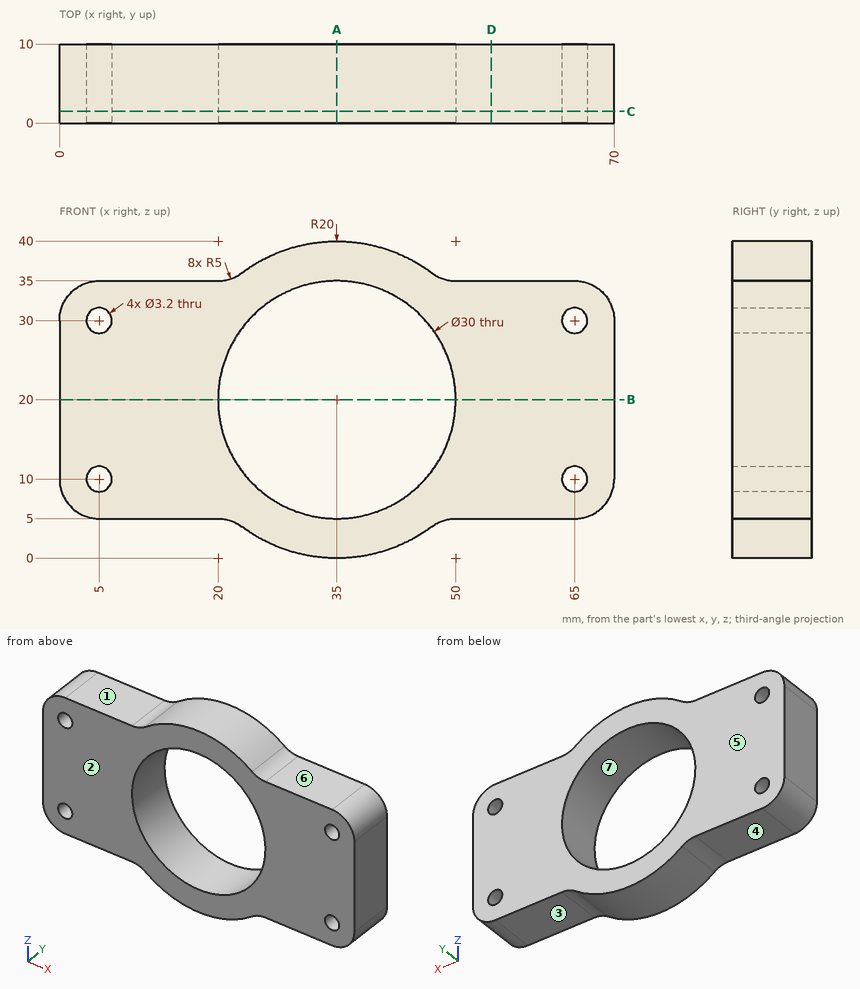
Input: dimensioned drawing with shaded views. Units: mm. Origin: part minimum x, y, z. A direction names the side the tool comes from. Coordinates: 2 decimals unless noted, no trailing zeros. Order: outer loops, then holes, each group sorted by start corner. A loop starts at its lowest first (then second) coordinate and runs counter-clockwise, first axis right, second up. Notation, with made-up numbers: (86, 71) - (143, 71) arc R30 ccw to (143, 104) - close; hole circle Ø11 at (59, 21.25). An arc over 180 degrees is marked (long way). One line per item, written item: value.
1) Reachability of the marked faces 1, 2 and 3 from +Z, -Z, +X, -X, +Y, -Y: full face, straight path, thin tool, end or side. Return the list, or none.
Computed values:
face 1: +Z, -X, +Y, -Y
face 2: +Z, -Z, +X, -X, -Y
face 3: -Z, +X, +Y, -Y
2) Contact query for a flat-ended pin moving along its axis: pin 1 (5 mm diameter, centred on x = 10.5, y = 5.5, fed in from +Z). Output: stop coordinate, or through.
Computed values:
pin 1: stops at z = 35
3) Cut plane D-D on x = 54.5. Output: boundary loops of the cut face in (y, z).
Computed values:
outline: (0, 5) - (10, 5) - (10, 35) - (0, 35) - close
4) Cut plane B-B on z = 20. Output: boundary loops of the cut face in (x, y).
Computed values:
outline: (0, 0) - (20, 0) - (20, 10) - (0, 10) - close; (50, 0) - (70, 0) - (70, 10) - (50, 10) - close
5) Mould query, pull axis Z, two halves, no side actions, for the marked faces 4, 5, 6 and 7. Classes: released by +Z, released by -Z, zero draft, split by the parting line, or undercut.
Computed values:
face 4: released by -Z
face 5: zero draft
face 6: released by +Z
face 7: undercut
6) Ray query, line 1 (X direction, y = 5.75, z = 10); line 2 (Z direction, x = 5, y = 3.5); line 3 (X direction, y = 2.75, z = 20). Return the intervals inside material, ascending. Write a range as [from, to].
Computed values:
line 1: x = [0, 3.4], [6.6, 23.82], [46.18, 63.4], [66.6, 70]
line 2: z = [5, 8.4], [11.6, 28.4], [31.6, 35]
line 3: x = [0, 20], [50, 70]
7) Cut plane C-C on y = 1.5. Output: boundary loops of the cut face in (x, z), plus the area to 3 significant figures.
Computed values:
outline: (0, 10) arc R5 ccw to (5, 5) - (20, 5) arc R5 cw to (23, 4) arc R20 ccw to (47, 4) arc R5 cw to (50, 5) - (65, 5) arc R5 ccw to (70, 10) - (70, 30) arc R5 ccw to (65, 35) - (50, 35) arc R5 cw to (47, 36) arc R20 ccw to (23, 36) arc R5 cw to (20, 35) - (5, 35) arc R5 ccw to (0, 30) - close; hole circle Ø3.2 at (5, 10); hole circle Ø3.2 at (5, 30); hole circle Ø30 at (35, 20); hole circle Ø3.2 at (65, 10); hole circle Ø3.2 at (65, 30)
area: 1,520 mm^2
8) Cut plane A-A on x = 35. Output: boundary loops of the cut face in (y, z), plus the area to 3 significant figures.
Computed values:
outline: (0, 0) - (10, 0) - (10, 5) - (0, 5) - close; (0, 35) - (10, 35) - (10, 40) - (0, 40) - close
area: 100 mm^2
